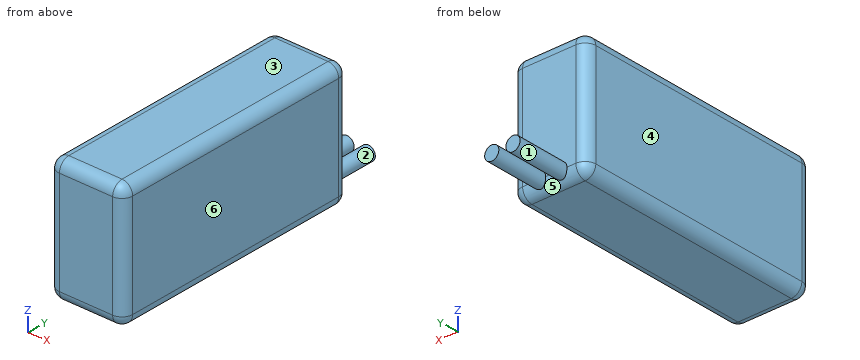
Autodesk Inventor part; units mm, degrees
ref_plane "YZ Plane" through (0, 0, 0) normal (1, 0, 0) x (0, 1, 0)
ref_plane "XZ Plane" through (0, 0, 0) normal (0, 1, 0) x (-1, 0, 0)
ref_plane "XY Plane" through (0, 0, 0) normal (0, 0, 1) x (1, 0, 0)
sketch "Sketch1" plane through (0, 0, 0) normal (0, 1, 0) x (-1, 0, 0)
  line L0 (10.5, 17.5) -> (-10.5, 17.5)
  line L1 (-10.5, 17.5) -> (-10.5, -17.5)
  line L2 (-10.5, -17.5) -> (10.5, -17.5)
  line L3 (10.5, -17.5) -> (10.5, 17.5)
  line L4 (10.5, 17.5) -> (-10.5, -17.5) construction
  line L5 (-10.5, 17.5) -> (10.5, -17.5) construction
  line L6 (0, -17.5) -> (0, -14.5) construction
  line L7 (0, -14.5) -> (3, -14.5) construction
  circle A0 centre (3, -14.5) radius 2
  circle A1 centre (-3, -14.5) radius 2
  point P0 (0, 0)
  dimension "d0" = 21
  dimension "d1" = 35
  dimension "d5" = 3
  dimension "d6" = 3
  dimension "d7" = 4
extrude "Extrusion1" add sketch "Sketch1" along normal blind 72 contours L3 L2 L1 L0 | A0 | A1
extrude "Extrusion2" add sketch "Sketch1" along normal blind 15 from surface at 72 contours A0 | A1
fillet "Fillet1" radius 3 12 edges at (10.5, 36, 17.5) (10.5, 36, -17.5) (-10.5, 36, 17.5) (-10.5, 36, -17.5) (10.5, 72, 0) (0, 72, 17.5) (0, 72, -17.5) (-10.5, 72, 0) (10.5, 0, 0) (0, 0, 17.5) (-10.5, 0, 0) (0, 0, -17.5)
properties part number "SLS X-CUBE 1250mAh 3S1P 11,1V 60"
Read the model definition and answer for the solid it produces. Units are mm, in the model's axes. Face numbers are marked on the shaded views. A direction names the side the tool comes from. Round coordinates to 2 decimals unless told otherwise and drop trailing zeros. Write each loop counter-clockwise with the first axis right and the second up, starting at its lowest first coordinate (ties: lowest second). Pieces come first, ordered by that corner, then holes. Notation, with made-up numbers: (74, 17) - (110, 17) arc R19 ccw to (110, 36) - close; hole circle Ø7 at (49.25, -23). An arc over 180 degrees is marked (long way). Use a Markdown table: item, result.
(1) Straight lines are drawn through the part: line 1 along Y through (x, z) = (4, 10.5); line 2 along Z through (x, y) = (-3.25, 80); line 3 along X through (y, z) = (19.5, 15). For each, find the intervals that lie inside material, in ascending order. Write a range as [from, to].
Reported:
| item | result |
|---|---|
| line 1 | [0, 72] |
| line 2 | [-16.48, -12.52] |
| line 3 | [-10.46, 10.46] |
(2) The part is cut by section C-C (z = 6.5). Write down the section's boundary in (x, y).
Reported:
| item | result |
|---|---|
| outline | (-10.5, 3) arc R3 ccw to (-7.5, 0) - (7.5, 0) arc R3 ccw to (10.5, 3) - (10.5, 69) arc R3 ccw to (7.5, 72) - (-7.5, 72) arc R3 ccw to (-10.5, 69) - close |
(3) The mould has two halves that part along X. Classify the marked faces 1, 2, 3 and 4: released by +X, released by -X, zero draft, split by the parting line, or undercut.
Reported:
| item | result |
|---|---|
| face 1 | undercut |
| face 2 | undercut |
| face 3 | zero draft |
| face 4 | released by -X |
(4) The part is cut by section B-B (y = 74). Write down the section's boundary in (x, z), then the cut area to 3 significant figures.
Reported:
| item | result |
|---|---|
| outline | circle Ø4 at (-3, -14.5); circle Ø4 at (3, -14.5) |
| area | 25.1 mm2 |
(5) The part is cut by section A-A (x = -3). Write down the section's boundary in (y, z).
Reported:
| item | result |
|---|---|
| outline | (0, -14.5) arc R3 ccw to (3, -17.5) - (69, -17.5) arc R3 ccw to (71.24, -16.5) - (87, -16.5) - (87, -12.5) - (72, -12.5) - (72, 14.5) arc R3 ccw to (69, 17.5) - (3, 17.5) arc R3 ccw to (0, 14.5) - close |
(6) The part is cut by section D-D (x = 6). Write down the section's boundary in (y, z), then the cut area to 3 significant figures.
Reported:
| item | result |
|---|---|
| outline | (0, -14.5) arc R3 ccw to (3, -17.5) - (69, -17.5) arc R3 ccw to (72, -14.5) - (72, 14.5) arc R3 ccw to (69, 17.5) - (3, 17.5) arc R3 ccw to (0, 14.5) - close |
| area | 2,510 mm2 |
(7) Each of these flat-tipped pins is pushed along its axis until it touches: pin 1 Ø4 at (x, z) = (-4.5, -2) entering from +Y; pin 2 Ø6 at (x, y) = (-8, 26.5) entering from +Z. Where does it stop, or does it pass through?
Reported:
| item | result |
|---|---|
| pin 1 | y = 72 |
| pin 2 | z = 17.5 |
(8) Which of the six approach directions +Z, -Z, +X, -X, +Y, -Y give full straight-line access (tool end or side, diameter ignored) to the marked faces 5 and 6?
Reported:
| item | result |
|---|---|
| face 5 | -Z, +Y |
| face 6 | +Z, -Z, +X, +Y, -Y |
